Model file for the job. Use its own axes, mm. Give positions to 0.01 mm unless a question says otherwise; leave off trailing zeros. Order: outer loops, then holes, each group sorted by start corner. A loop starts at its lowest first (then second) coordinate and runs counter-clockwise, first axis right, second up. Notation, with made-up numbers: M 31,35.25 L 84,35.25 A24 ccw 84,51.25 Z; hole C -26.5,84 d3. An arc over 180 degrees is marked long. Return JSON: item names as keys, results as strings. Group by question number.
1. Slice it at D-D on z = 78.5. List the corners of the cut face in (x, y), then the cut area to 3 significant figures.
2. Wall check: probe 1 along Z at (x, y) = (0, 1.25); probe 2 along Y at (x, z) = (67, 111); probe 3 along Z at (x, y) = (-30.5, -1). Give the ranges that are in metal, low to high. Write a range as [from, to].
3. Slice it at A-A on z = 0. List the corners of the cut face in (x, y), then the cut area to 3 significant figures.
4. Slice it at C-C on x = -84.5. List the corners of the cut face in (y, z), then the cut area to 3 significant figures.
5. Pin check, flat tips, straight feed: pin 1 (2 mm diameter, centred on x = 80.5, z = 148, fed in from -Y); pin 2 (12 mm diameter, centred on x = -116.67, z = 116.67, fed in from +Y); pin 3 (8 mm diameter, centred on x = -15, z = 117.5, fed in from -Y); pin 4 (1.6 mm diameter, centred on y = 1.5, z = 16.5, fed in from +X). Stop position of each tip, or through.
6. Slice it at B-B on x = 0. List the corners of the cut face in (y, z), then the cut area to 3 significant figures.
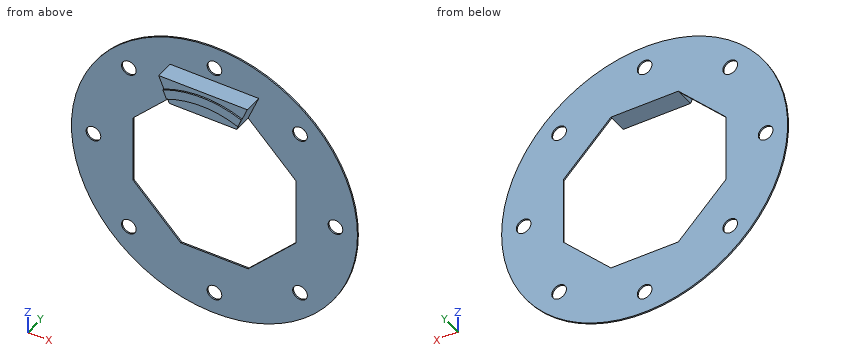
from build123d import *

# Parameters (mm, degrees)
F1_DEPTH = 25
F3_DEPTH = 2
F4_R     = 195
F4_R_2   = 10
F5_DEPTH = 2


with BuildPart() as f1:
    # F0 (on Front) → F1 (new body)
    with BuildSketch(Plane.XZ):
        Polygon((-60.394094, 145.804241), (-45.933053, 110.892201), (45.933053, 110.892201), (60.394094, 145.804241), align=None)
    extrude(amount=F1_DEPTH)

    # F2 (on face) → F3 (join)
    with BuildSketch(Plane.XZ.offset(25)):
        with BuildLine():
            Line((-53.460876, 129.065971), (-48.600796, 117.332701))
            ThreePointArc((-48.600796, 117.332701), (0, 127), (48.600796, 117.332701))
            Line((48.600796, 117.332701), (53.460876, 129.065971))
            ThreePointArc((53.460876, 129.065971), (0, 139.7), (-53.460876, 129.065971))
        make_face()
    extrude(amount=F3_DEPTH)

    # F4 (on face) → F5 (join)
    with BuildSketch(Plane.XZ):
        Circle(F4_R)
        with Locations((-116.672619, -116.672619)):
            Circle(F4_R_2, mode=Mode.SUBTRACT)
        with Locations((0, -165)):
            Circle(F4_R_2, mode=Mode.SUBTRACT)
        with Locations((116.672619, -116.672619)):
            Circle(F4_R_2, mode=Mode.SUBTRACT)
        with Locations((-165, 0)):
            Circle(F4_R_2, mode=Mode.SUBTRACT)
        with Locations((-116.672619, 116.672619)):
            Circle(F4_R_2, mode=Mode.SUBTRACT)
        Polygon((-110.892201, -45.933053), (-110.892201, 45.933053), (-45.933053, 110.892201), (45.933053, 110.892201), (110.892201, 45.933053), (110.892201, -45.933053), (45.933053, -110.892201), (-45.933053, -110.892201), align=None, mode=Mode.SUBTRACT)
        with Locations((165, 0)):
            Circle(F4_R_2, mode=Mode.SUBTRACT)
        with Locations((0, 165)):
            Circle(F4_R_2, mode=Mode.SUBTRACT)
        with Locations((116.672619, 116.672619)):
            Circle(F4_R_2, mode=Mode.SUBTRACT)
    extrude(amount=-F5_DEPTH)


solid = f1.part
Result:
{
 "1": {"outline": "M -178.5,0 L -78.33,0 L -78.33,2 L -178.5,2 Z; M 78.33,0 L 178.5,0 L 178.5,2 L 78.33,2 Z", "area": "401 mm2"},
 "2": {"probe 1": "z = [-195, -175], [-155, -110.89], [110.89, 155], [175, 195]", "probe 2": "y = [0, 2]", "probe 3": "z = [110.89, 145.8]"},
 "3": {"outline": "M -195,0 L -175,0 L -175,2 L -195,2 Z; M -155,0 L -110.89,0 L -110.89,2 L -155,2 Z; M 110.89,0 L 155,0 L 155,2 L 110.89,2 Z; M 175,0 L 195,0 L 195,2 L 175,2 Z", "area": "256 mm2"},
 "4": {"outline": "M 0,-175.74 L 2,-175.74 L 2,-72.33 L 0,-72.33 Z; M 0,72.33 L 2,72.33 L 2,175.74 L 0,175.74 Z", "area": "414 mm2"},
 "5": {"pin 1": "stops at y = 0", "pin 2": "passes through", "pin 3": "stops at y = -25", "pin 4": "stops at x = 194.37"},
 "6": {"outline": "M -27,127 L -25,127 L -25,110.89 L 2,110.89 L 2,155 L 0,155 L 0,145.8 L -25,145.8 L -25,139.7 L -27,139.7 Z; M 0,-195 L 2,-195 L 2,-175 L 0,-175 Z; M 0,-155 L 2,-155 L 2,-110.89 L 0,-110.89 Z; M 0,175 L 2,175 L 2,195 L 0,195 Z", "area": "1,150 mm2"}
}
